Geometry: final body of the model. Coordinates: model frame, mm. Give positions to 0.01 mm unless a question says otherwise; leave off trailing zeros. Loops run counter-clockwise (first coordinate to the right, second up) from the corner with the lowest first, then second, coordinate; pieces in that order, holes last.
1. Section A-A, the plane z = 72. Output: boundary loops of the cut face in (x, y), then the cut area to 3 significant figures.
2. First-contact query: P1, Ø1.5, axis at y = 1, z = 39, coming from the +X side; P2, Ø1.5, axis at y = 4, z = 53.5, coming from the -X side; P3, Ø2, axis at x = -2.5, y = -2, coming from the +Z side. Flat tips, straight axial feed; report the tip coordinate or a pass-through.
3. Material intervals for line 1 along Y through (x, z) = (0, 47); line 2 along X through (y, z) = (-0.5, 32), sorted ascending.
4. Draft query along X for faces 1 (the face through (-0.74, -3.32, 34)), 2 (the face through (-1.08, -4.88, 72.9)). Return one class per face: +X half, -X half, draft (parallel to the pull), parting line (faces both ways), or undercut.
5. Section B-B, the plane z = 13. Output: boundary loops of the cut face in (x, y).
from build123d import *

# Parameters (mm, degrees)
SKETCH_1_R             = 5
EXTRUDE_1_DEPTH        = 80.5
PATTERN_LINEAR_1_COUNT = 2
PATTERN_LINEAR_1_PITCH = 30
HOLE_WIZARD_M8_1_D     = 6.8
HOLE_WIZARD_M8_1_DEPTH = 67.07
HOLE_WIZARD_M8_1_TIP   = 1.962990915


with BuildPart() as part:
    # 草图1 → 凸台-拉伸1 (new body)
    with BuildSketch(Plane.XY):
        Circle(SKETCH_1_R)
    extrude(amount=EXTRUDE_1_DEPTH)

    # 草图2 → 切除-旋转1 (revolve, cut)
    with BuildSketch(Plane(origin=(0, 0, 0), x_dir=(0, 0, -1), z_dir=(1, 0, 0)), mode=Mode.PRIVATE) as cut_revolve_1_sk:
        Polygon((-28.5, 5), (-29, 4.5), (-29.5, 5), align=None)
    cut_revolve_1 = revolve(cut_revolve_1_sk.sketch.rotate(Axis((0, 0, 95.745641227), (0, 0, -1)), 90), axis=Axis((0, 0, 95.745641227), (0, 0, -1)), mode=Mode.SUBTRACT)

    # 草图4 → 切除-旋转2 (revolve, cut)
    with BuildSketch(Plane(origin=(0, 0, 0), x_dir=(0, 0, -1), z_dir=(1, 0, 0)), mode=Mode.PRIVATE) as cut_revolve_2_sk:
        Polygon((-31.5, 5), (-32, 4.5), (-32.5, 5), align=None)
        Polygon((-34.5, 5), (-35, 4.5), (-35.5, 5), align=None)
    cut_revolve_2 = revolve(cut_revolve_2_sk.sketch.rotate(Axis((0, 0, -1.972626415), (0, 0, 1)), 90), axis=Axis((0, 0, -1.972626415), (0, 0, 1)), mode=Mode.SUBTRACT)

    # 阵列(线性)1: 切除-旋转1, 切除-旋转2 ×2
    with Locations(*[(0, 0, i * PATTERN_LINEAR_1_PITCH) for i in range(1, PATTERN_LINEAR_1_COUNT)]):
        add(cut_revolve_1, mode=Mode.SUBTRACT)
        add(cut_revolve_2, mode=Mode.SUBTRACT)

    # 草图5 → 旋转2 (revolve)
    with BuildSketch(Plane(origin=(0, 0, 0), x_dir=(0, 0, -1), z_dir=(1, 0, 0)), mode=Mode.PRIVATE) as revolve_2_sk:
        with BuildLine():
            Line((-80.5, 5), (-80.5, 0))
            Line((-80.5, 0), (-85, 0))
            add(Edge.make_bspline(
                [(-80.5, 5), (-81.808902232, 4.887546308), (-83.760685611, 3.318595148), (-84.908352583, 1.178697403), (-85, 0)],
                knots=[0, 0, 0, 0, 0.52200898, 1, 1, 1, 1], degree=3))
        make_face()
    revolve(revolve_2_sk.sketch.rotate(Axis((0, 0, 87.782786163), (0, 0, -1)), 270), axis=Axis((0, 0, 87.782786163), (0, 0, -1)))

    # M8 螺纹孔1
    with Locations(Plane(origin=(0, 0, 0), x_dir=(-1, 0, 0), z_dir=(0, 0, -1))):
        with Locations((0, 0)):
            Hole(HOLE_WIZARD_M8_1_D / 2, depth=HOLE_WIZARD_M8_1_DEPTH)
            with Locations((0, 0, -(HOLE_WIZARD_M8_1_DEPTH + HOLE_WIZARD_M8_1_TIP / 2))):  # 120° drill point
                Cone(0, HOLE_WIZARD_M8_1_D / 2, HOLE_WIZARD_M8_1_TIP, mode=Mode.SUBTRACT)


solid = part.part
Answers below:
1. outline: circle Ø10 at (0, 0)
1. area: 78.5 mm2
2. P1: stops at x = 4.99
2. P2: stops at x = -3.8
2. P3: stops at z = 84.26
3. line 1: y = -5 to -3.4, 3.4 to 5
3. line 2: x = -4.47 to -3.36, 3.36 to 4.47
4. face 1: undercut
4. face 2: parting line
5. outline: circle Ø10 at (0, 0); hole circle Ø6.8 at (0, 0)
